```python
from build123d import *

# Parameters (mm, degrees)
SKETCH2_R           = 4.566933549
BOSS_EXTRUDE1_DEPTH = 10
SKETCH3_W           = 42.436263922
SKETCH3_H           = 22.27820436
BOSS_EXTRUDE2_DEPTH = 20
RIB2_REACH          = 66.498
SKETCH5_WALL_W      = 166.044941872
SKETCH5_WALL_H      = 4
BOSS_EXTRUDE3_DEPTH = 2
SKETCH7_R           = 11.13910218
SKETCH7_R_2         = 6.13910218
EXTRUDE_THIN1_DEPTH = 9
SKETCH9_R           = 6.13910218
CUT_EXTRUDE2_DEPTH  = 65.498231097
SKETCH12_R          = 10
CUT_EXTRUDE4_DEPTH  = 19
CUT_EXTRUDE4_DRAFT  = -11.5
SKETCH13_W          = 13.380488588
SKETCH13_H          = 1.799910433
CUT_EXTRUDE5_DEPTH  = 9


with BuildPart() as part:
    # Sketch2 → Boss-Extrude1 (new body)
    with BuildSketch(Plane(origin=(0, 0, 0), x_dir=(1, 0, 0), z_dir=(0, 1, 0))):
        with BuildLine():
            Line((-50, 20), (-18.974240817, 20))
            ThreePointArc((-18.974240817, 20), (0, 27.568493151), (18.974240817, 20))
            Line((18.974240817, 20), (50, 20))
            Line((50, 20), (50, -20))
            Line((50, -20), (18.974240817, -20))
            ThreePointArc((18.974240817, -20), (0, -27.568493151), (-18.974240817, -20))
            Line((-18.974240817, -20), (-50, -20))
            Line((-50, -20), (-50, 20))
        make_face()
        with Locations(Location((-40.274600864, 11.13910218, 0), (0, 0, 270))):
            Circle(SKETCH2_R, mode=Mode.SUBTRACT)
        with Locations(Location((-40.274600864, -11.13910218, 0), (0, 0, 90))):
            Circle(SKETCH2_R, mode=Mode.SUBTRACT)
        with Locations(Location((40.274600864, -11.13910218, 0), (0, 0, 270))):
            Circle(SKETCH2_R, mode=Mode.SUBTRACT)
        with Locations(Location((40.274600864, 11.13910218, 0), (0, 0, 90))):
            Circle(SKETCH2_R, mode=Mode.SUBTRACT)
    extrude(amount=BOSS_EXTRUDE1_DEPTH)

    # Sketch3 → Boss-Extrude2 (add)
    with BuildSketch(Plane(origin=(0, 10, 0), x_dir=(1, 0, 0), z_dir=(0, 1, 0))):
        Rectangle(SKETCH3_W, SKETCH3_H)
    extrude(amount=BOSS_EXTRUDE2_DEPTH)

    # Sketch5 wall → Rib2 (add, up to next)
    with BuildSketch(Plane(origin=(-35.60906598, 20, 0), x_dir=(-0.82120161281, -0.570638161288, 0), z_dir=(0.570638161288, -0.82120161281, 0)), mode=Mode.PRIVATE) as rib2_sk1:
        Rectangle(SKETCH5_WALL_W, SKETCH5_WALL_H)
    rib2_tool1 = extrude(rib2_sk1.sketch, amount=RIB2_REACH, mode=Mode.PRIVATE) - part.part
    add(rib2_tool1.solids().sort_by_distance((-35.60906598, 20, 0))[0])

    # Sketch6 → Boss-Extrude3 (add, symmetric)
    with BuildSketch(Plane.XY):
        Polygon((21.218131961, 30), (50, 10), (21.218131961, 10), align=None)
    extrude(amount=BOSS_EXTRUDE3_DEPTH, both=True)

    # Sketch7 → Extrude-Thin1 (add)
    with BuildSketch(Plane(origin=(0, 30, 0), x_dir=(1, 0, 0), z_dir=(0, 1, 0))):
        Circle(SKETCH7_R)
        Circle(SKETCH7_R_2, mode=Mode.SUBTRACT)
    extrude(amount=EXTRUDE_THIN1_DEPTH)

    # Sketch9 → Cut-Extrude2 (cut, through all)
    with BuildSketch(Plane(origin=(0, 30, 0), x_dir=(1, 0, 0), z_dir=(0, 1, 0))):
        Circle(SKETCH9_R)
    extrude(amount=-CUT_EXTRUDE2_DEPTH, mode=Mode.SUBTRACT)


with BuildPart() as cut_extrude4_tool:
    # Sketch12 → Cut-Extrude4 (with draft: the straight prism first)
    with BuildSketch(Plane.XZ):
        Circle(SKETCH12_R)
    extrude(amount=-CUT_EXTRUDE4_DEPTH)
    # Cut-Extrude4: the draft: its side faces are tilted about the plane it starts from
    cut_extrude4_sides = [cut_extrude4_tool.faces().sort_by_distance(p)[0] for p in [
        (-10, 9.5, 0),
    ]]
    draft(cut_extrude4_sides, Plane.XZ, CUT_EXTRUDE4_DRAFT)


with BuildPart() as part_1:
    add(part.part)

    # Cut-Extrude4: cut by cut_extrude4_tool
    add(cut_extrude4_tool.part, mode=Mode.SUBTRACT)

    # Sketch13 → Cut-Extrude5 (cut)
    with BuildSketch(Plane.XY.offset(11.13910218)):
        with Locations((0, 26.881553508)):
            Rectangle(SKETCH13_W, SKETCH13_H)
    extrude(amount=-CUT_EXTRUDE5_DEPTH, mode=Mode.SUBTRACT)


solid = part_1.part
```
Design review of the part built by this model. Coordinates are the model's own, in mm. A direction names the side the tool comes from. Round coordinates to 2 decimals unless told otherwise and drop trailing zeros. Order: outer loops, then holes, each group sorted by start corner. A loop starts at its lowest first (then second) coordinate and runs counter-clockwise, first axis right, second up. Notation, with made-up numbers: (1.5, -5) - (11.5, -5) arc R20 cw to (11.5, 18) - close; hole circle Ø5 at (17.5, -30.75). An arc over 180 degrees is marked (long way). One line per question, with ' | ' between items.
Item 1: Take a section at D-D, the plane y = 5. Write out the cut boundary in (x, z), then the cut area to 3 significant figures.
Checks:
outline: (-50, -20) - (-18.97, -20) arc R27.57 ccw to (18.97, -20) - (50, -20) - (50, 20) - (18.97, 20) arc R27.57 ccw to (-18.97, 20) - (-50, 20) - close; hole circle Ø9.13 at (-40.27, -11.14); hole circle Ø9.13 at (-40.27, 11.14); hole circle Ø17.97 at (0, 0); hole circle Ø9.13 at (40.27, -11.14); hole circle Ø9.13 at (40.27, 11.14) | area: 3,880 mm²
Item 2: Take a section at C-C, the plane x = -30. Write out the cut boundary in (y, z).
Checks:
outline: (0, -20) - (10, -20) - (10, -2) - (23.9, -2) - (23.9, 2) - (10, 2) - (10, 20) - (0, 20) - close
Item 3: Machinability: for faces 4 (the face through (1, 10, 12)), 5 (the face through (34, 5, -20)), 6 (the face through (-21.218, 20, 7)), which of the approach directions +Z, -Z, +X, -X, +Y, -Y give a long, thin tool a straight path to every point of the face, cutting with its end or side? Answer none if there is none.
Checks:
face 4: +Z, +Y | face 5: -Z, +X, +Y, -Y | face 6: +Z, -X, +Y
Item 4: Wall thickness on line 1 (Z direction, x = 0, y = 23.5); line 2 (X direction, y = 14, z = 2.5): over which ranges is each line inside the solid? List them lowest first. Write a range as [from, to].
Checks:
line 1: [-11.14, -6.14], [6.14, 11.14] | line 2: [-21.22, -6.7], [6.7, 21.22]
Item 5: Draft analysis for pull direction Y (two halves, no side actions). For faces 1 (the face through (0.293, 4.93, 27.567)), 2 (the face through (35.41, 20.14, 0.03)), 3 (the face through (0, 27.782, 8)), state which applies: +Y half, -Y half, draft (parallel to the pull), parting line (faces both ways), or undercut.
Checks:
face 1: draft | face 2: +Y half | face 3: undercut
Item 6: Take a section at A-A, the plane z = 0. Write out the cut boundary in (x, y).
Checks:
outline: (-50, 0) - (-10, 0) - (-6.14, 18.98) - (-6.14, 39) - (-11.14, 39) - (-11.14, 30) - (-21.22, 30) - (-50, 10) - close; (6.14, 18.98) - (10, 0) - (50, 0) - (50, 10) - (21.22, 30) - (11.14, 30) - (11.14, 39) - (6.14, 39) - close
Item 7: For P1, Ø11, axis at x = 38, y = 3.5, coming from the -Z side; P2, Ø2.5, axis at y = 19.5, z = -7.5, coming from the -X side; P3, Ø22, axis at x = 33, y = 22, coming from the +Z side; P4, Ø10, axis at x = 0, z = 0, coming from the +Y side, all flat-tipped, find the tip position at first contact; note any pin that passes through.
Checks:
P1: z = -20 | P2: x = -21.22 | P3: z = 2 | P4: through
Item 8: Take a section at B-B, the plane y = 14. Write out the cut boundary in (x, z), then the cut area to 3 significant figures.
Checks:
outline: (-44.24, -2) - (-21.22, -2) - (-21.22, -11.14) - (21.22, -11.14) - (21.22, -2) - (44.24, -2) - (44.24, 2) - (21.22, 2) - (21.22, 11.14) - (-21.22, 11.14) - (-21.22, 2) - (-44.24, 2) - close; hole circle Ø14.3 at (0, 0) | area: 969 mm²
